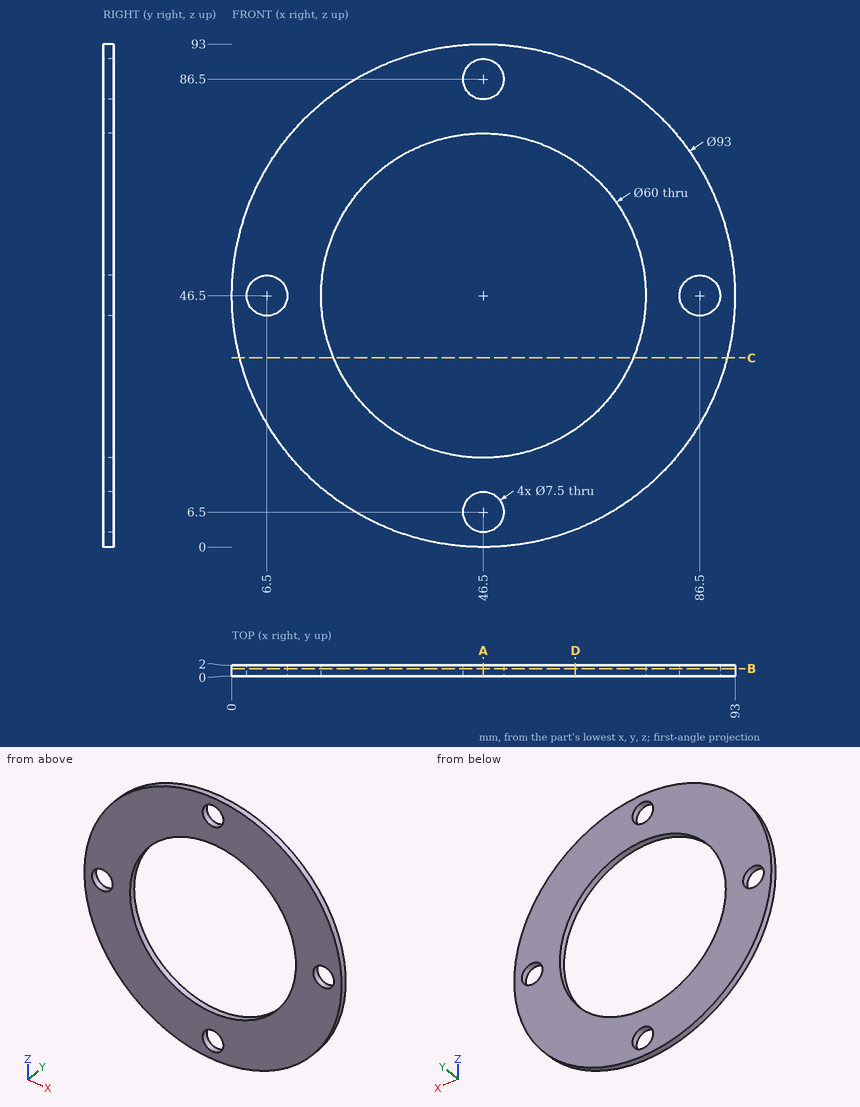
Can you work these out from the drawing? Everything is in mm from the part's minimum corner. Coordinates: 2 decimals unless noted, no trailing zeros. Loops run counter-clockwise (first coordinate to the right, second up) from the corner with the lowest first, then second, coordinate; pieces in that order, holes last.
1) Imagine slicing it at D-D on x = 63.5. List the corners of the cut face in (y, z) for me.
2) Imagine slicing it at A-A on x = 46.5. List the corners of the cut face in (y, z) for me.
3) Imagine slicing it at B-B on y = 1.35. List the corners of the cut face in (x, z) for me.
4) I need wall thicknesses on probe 1 along Z at (x, y) = (46.5, 0.55); probe 2 along Z at (x, y) = (44, 0.55); probe 3 along Z at (x, y) = (6.5, 1.1). Which ranges of each line are inside material? Lowest first, please.
5) For pin 1 (10 mm diameter, centred on x = 86.5, z = 46.5, fed in from -Y); pin 2 (10 mm diameter, centred on x = 52.5, z = 23.5, fed in from +Y), each with a flat end and sliding along its axis, tell me the tip position at first contact or that it passes through.
6) Imagine slicing it at C-C on z = 35. List the corners of the cut face in (x, y) for me.
Completed:
1. outline: (0, 3.22) - (2, 3.22) - (2, 21.78) - (0, 21.78) - close; (0, 71.22) - (2, 71.22) - (2, 89.78) - (0, 89.78) - close
2. outline: (0, 0) - (2, 0) - (2, 2.75) - (0, 2.75) - close; (0, 10.25) - (2, 10.25) - (2, 16.5) - (0, 16.5) - close; (0, 76.5) - (2, 76.5) - (2, 82.75) - (0, 82.75) - close; (0, 90.25) - (2, 90.25) - (2, 93) - (0, 93) - close
3. outline: circle Ø93 at (46.5, 46.5); hole circle Ø7.5 at (6.5, 46.5); hole circle Ø60 at (46.5, 46.5); hole circle Ø7.5 at (46.5, 6.5); hole circle Ø7.5 at (46.5, 86.5); hole circle Ø7.5 at (86.5, 46.5)
4. probe 1: z = 0 to 2.75, 10.25 to 16.5, 76.5 to 82.75, 90.25 to 93
4. probe 2: z = 0.07 to 3.7, 9.3 to 16.6, 76.4 to 83.7, 89.3 to 92.93
4. probe 3: z = 22.79 to 42.75, 50.25 to 70.21
5. pin 1: stops at y = 0
5. pin 2: passes through
6. outline: (1.44, 0) - (18.79, 0) - (18.79, 2) - (1.44, 2) - close; (74.21, 0) - (91.56, 0) - (91.56, 2) - (74.21, 2) - close
